from build123d import *

# Parameters (mm, degrees)
F0_W     = 23
F0_H     = 28
F0_W_2   = 19
F0_H_2   = 24
F0_W_3   = 15
F0_H_3   = 20
F1_DEPTH = 2
F2_DEPTH = 25
F3_DEPTH = 30
F4_W     = 12
F4_H     = 3
F5_DEPTH = 5
F6_W     = 11
F6_H     = 2
F7_DEPTH = 2


with BuildPart() as f1:
    # F0 (on Top) → F1 (new body)
    with BuildSketch(Plane.XY):
        Rectangle(F0_W, F0_H)
        Rectangle(F0_W_2, F0_H_2, mode=Mode.SUBTRACT)
        Rectangle(F0_W_2, F0_H_2)
        Rectangle(F0_W_3, F0_H_3, mode=Mode.SUBTRACT)
        Rectangle(F0_W_3, F0_H_3)
    extrude(amount=F1_DEPTH)

    # F0 (on Top) → F2 (cut)
    with BuildSketch(Plane.XY):
        Rectangle(F0_W_3, F0_H_3)
    extrude(amount=F2_DEPTH, mode=Mode.SUBTRACT)

    # F0 (on Top) → F3 (join)
    with BuildSketch(Plane.XY):
        Rectangle(F0_W, F0_H)
        Rectangle(F0_W_2, F0_H_2, mode=Mode.SUBTRACT)
    extrude(amount=F3_DEPTH)

    # F4 (on face) → F5 (cut)
    with BuildSketch(Plane(origin=(0, 14, 0), x_dir=(-1, 0, 0), z_dir=(0, 1, 0))):
        with Locations((0, 26.5)):
            Rectangle(F4_W, F4_H)
    extrude(amount=-F5_DEPTH, mode=Mode.SUBTRACT)

    # F6 (on face) → F7 (join)
    with BuildSketch(Plane(origin=(0, -12, 0), x_dir=(-1, 0, 0), z_dir=(0, 1, 0))):
        with Locations((0, 26.5)):
            Rectangle(F6_W, F6_H)
    extrude(amount=F7_DEPTH)


solid = f1.part
Can you work these out from the model? Positions are in its coordinate system, mm. A direction names the side the tool comes from. Coordinates: 2 decimals unless noted, no trailing zeros. Order: outer loops, then holes, each group sorted by start corner. A loop starts at its lowest first (then second) coordinate and runs counter-clockwise, first axis right, second up. Notation, with made-up numbers: M -19,-13 L 17,-13 A11 ccw 17,-7 Z; hole C 29.25,77.5 d5. An arc over 180 degrees is marked long. Answer as CSV lines item,"result".
(1) Suppose I cut it at A-A on x = -3.75. Please give me the cut outline in (y, z).
Geometry check:
outline,"M -14,0 L -10,0 L -10,2 L -12,2 L -12,25.5 L -10,25.5 L -10,27.5 L -12,27.5 L -12,30 L -14,30 Z; M 10,0 L 14,0 L 14,25 L 12,25 L 12,2 L 10,2 Z; M 12,28 L 14,28 L 14,30 L 12,30 Z"
(2) I'm going to push flat-ended pins straight in: pin 1 (1.6 mm diameter, centred on x = -0.5, y = -11, fed in from +Z); pin 2 (6 mm diameter, centred on x = 5.5, y = 8, fed in from +Z). Where does each tip first touch, or does it pass through?
Geometry check:
pin 1,"z = 27.5"
pin 2,"z = 2"
(3) Please list where these lines run through material, in increasing order: L1, parallel to X at y = 2.75, z = 4; L2, parallel to Y at x = -6, z = 21.75; L3, parallel to Z at x = 4.25, y = -11.
Geometry check:
L1,"-11.5 to -9.5, 9.5 to 11.5"
L2,"-14 to -12, 12 to 14"
L3,"0 to 2, 25.5 to 27.5"
(4) On a 3-axis mill with a long thin cutter (end or side, diameter ignored), from which of +Z, -Z, +X, -X, +Y, -Y can I reach the whole of each face in a straight line? I mean faces 5 (the flat face through (0, 12, 16)), 6 (the flat face through (0, -10, 27)), 7 (the flat face through (8, 0, 2)), 8 (the flat face through (0, -11, 27.5)), 9 (the flat face through (0, 10, 1)). Say none if no direction works.
Geometry check:
face 5,"+Z"
face 6,"+Z, -Z, +Y"
face 7,"none"
face 8,"+Z, +Y"
face 9,"+Z, -Z"
(5) If we mould it in two halves opening along X, with no side actions, what happens to faces 1 (the flat face through (5.5, -11, 26)), 2 (the flat face through (11.5, 0, 15)), 3 (the flat face through (-9.5, 0, 16)), 4 (the flat face through (-8, 0, 0))? For each: released by +X, released by -X, zero draft, split by the parting line, or undercut.
Geometry check:
face 1,"undercut"
face 2,"released by +X"
face 3,"undercut"
face 4,"zero draft"
(6) Suppose I cut it at B-B on y = 1.5. Please give me the cut outline in (x, z).
Geometry check:
outline,"M -11.5,0 L -7.5,0 L -7.5,2 L -9.5,2 L -9.5,30 L -11.5,30 Z; M 7.5,0 L 11.5,0 L 11.5,30 L 9.5,30 L 9.5,2 L 7.5,2 Z"
(7) Suppose I cut it at C-C on x = 6.75. Please give me the cut outline in (y, z), plus the area to 3 significant figures.
Geometry check:
outline,"M -14,0 L -10,0 L -10,2 L -12,2 L -12,30 L -14,30 Z; M 10,0 L 14,0 L 14,30 L 12,30 L 12,2 L 10,2 Z"
area,"128 mm^2"
(8) Suppose I cut it at D-D on z = 16.5. Please give me the cut outline in (x, y).
Geometry check:
outline,"M -11.5,-14 L 11.5,-14 L 11.5,14 L -11.5,14 Z; hole M -9.5,-12 L 9.5,-12 L 9.5,12 L -9.5,12 Z"
